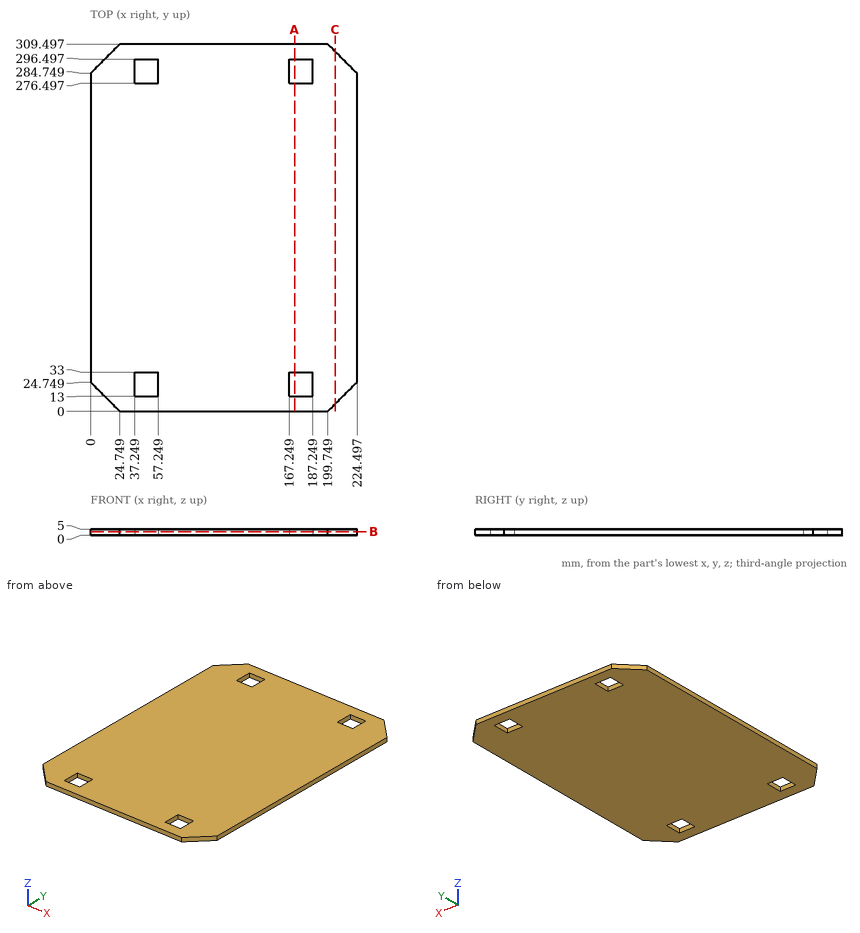
Geometry: see drawing. Coordinates: mm, zero at the bounding-box minimum. Coordinates: 2 decimals unless noted, no trailing zeros. Loops run counter-clockwise (first coordinate to the right, second up) from the corner with the lowest first, then second, coordinate; pieces in that order, holes last.
Q1. Contact query for a flat-ended pin moving along its axis: pin 1 (10 mm diameter, centred on x = 141, y = 158.5, fed in from -Z). Output: stop coordinate, or through.
Q2. Cut plane C-C (x = 206). Output: boundary loops of the cut face in (y, z).
Q3. Cut plane A-A (x = 172). Output: boundary loops of the cut face in (y, z).
Q4. Cut plane B-B (z = 3.2). Output: boundary loops of the cut face in (x, y).
Q5. Material intervals for line 1 (Y direction, x = 184, z = 4.25); line 2 (X direction, y = 14.5, z = 2.9); line 3 (Y direction, x = 16, z = 3.75), sorted ascending.
Working result:
1. pin 1: stops at z = 0
2. outline: (6.25, 0) - (303.25, 0) - (303.25, 5) - (6.25, 5) - close
3. outline: (0, 0) - (13, 0) - (13, 5) - (0, 5) - close; (33, 0) - (276.5, 0) - (276.5, 5) - (33, 5) - close; (296.5, 0) - (309.5, 0) - (309.5, 5) - (296.5, 5) - close
4. outline: (0, 24.75) - (24.75, 0) - (199.75, 0) - (224.5, 24.75) - (224.5, 284.75) - (199.75, 309.5) - (24.75, 309.5) - (0, 284.75) - close; hole (37.25, 13) - (57.25, 13) - (57.25, 33) - (37.25, 33) - close; hole (37.25, 276.5) - (57.25, 276.5) - (57.25, 296.5) - (37.25, 296.5) - close; hole (167.25, 13) - (187.25, 13) - (187.25, 33) - (167.25, 33) - close; hole (167.25, 276.5) - (187.25, 276.5) - (187.25, 296.5) - (167.25, 296.5) - close
5. line 1: y = 0 to 13, 33 to 276.5, 296.5 to 309.5
5. line 2: x = 10.25 to 37.25, 57.25 to 167.25, 187.25 to 214.25
5. line 3: y = 8.75 to 300.75
